The listing builds one solid part. Answer for the finished solid, in the listing's coordinates (mm). Face numbers are marked on the shaded views. A direction names the side the tool comes from. Round coordinates to 2 decimals unless told otherwise and drop trailing zeros. Write each loop counter-clockwise with the first axis right and the second up, starting at its lowest first coordinate (ties: lowest second). Pieces come first, ordered by that corner, then holes.
(1) Each of these flat-tipped pins is pushed along its axis until it touches: pin 1 Ø7.5 at (x, z) = (0, 0) entering from +Y; pin 2 Ø0.8 at (x, y) = (-10, 6) entering from +Z; pin 3 Ø0.8 at (y, z) = (5.5, 1) entering from -X; pin 4 Ø2 at (x, y) = (-7.5, 6) entering from -Z. Where does it stop, or does it pass through?
(2) A cutting plane is placed at C-C, the plane y = 2.75. Give the vertices of the cut face in (x, z) (3 decimals), and give its area (3 significant figures).
(3) A cutting plane is placed at A-A, the plane x = 0. Give the vertices of the cut face in (y, z) (3 decimals), and give its area (3 significant figures).
(4) Find the intervals of material crossed by probe 1 along X at (y, z) = (5.8, 0) (3 decimals); probe 2 along Z at (x, y) = (0, 5.3) (3 decimals); probe 3 along X at (y, z) = (4, -1), in increasing order.
(5) A cutting plane is placed at B-B, the plane z = 0. Give the vertices of the cut face in (x, y) (3 decimals), and give its area (3 significant figures).
(6) A cutting plane is placed at D-D, the plane z = -5.25. Give the vertices of the cut face in (x, y).
(7) For the marked faces 5, 6 and 7, determine the directions among +Z, -Z, +X, -X, +Y, -Y from which every point of the face is accessible in a straight line to the end or side of a thin tool.
(8) The mould has two halves that part along Z. Classify the marked faces 1, 2, 3 and 4: +Z half, -Z half, draft (parallel to the pull), parting line (faces both ways), or undercut.
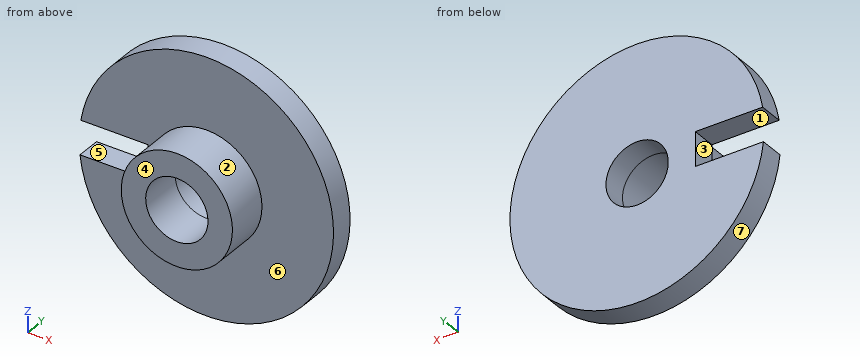
from build123d import *

# Parameters (mm, degrees)
SKETCH1_R           = 5.685
SKETCH1_R_2         = 3.185
BOSS_EXTRUDE1_DEPTH = 4.46
SKETCH2_R           = 13
BOSS_EXTRUDE2_DEPTH = 2.5
SKETCH3_R           = 3.185
CUT_EXTRUDE1_DEPTH  = 2.5
SKETCH4_W           = 8.515099108
SKETCH4_H           = 3.5
CUT_EXTRUDE2_DEPTH  = 10


with BuildPart() as part:
    # Sketch1 → Boss-Extrude1 (new body)
    with BuildSketch(Plane(origin=(0, 0, 0), x_dir=(1, 0, 0), z_dir=(0, 1, 0))):
        with Locations(Location((0, 0, 0), (0, 0, 270))):
            Circle(SKETCH1_R)
        with Locations(Location((0, 0, 0), (0, 0, 270))):
            Circle(SKETCH1_R_2, mode=Mode.SUBTRACT)
    extrude(amount=BOSS_EXTRUDE1_DEPTH)

    # Sketch2 → Boss-Extrude2 (add)
    with BuildSketch(Plane(origin=(0, 4.46, 0), x_dir=(1, 0, 0), z_dir=(0, 1, 0))):
        with Locations(Location((0, 0, 0), (0, 0, 270))):
            Circle(SKETCH2_R)
    extrude(amount=BOSS_EXTRUDE2_DEPTH)

    # Sketch3 → Cut-Extrude1 (cut)
    with BuildSketch(Plane.XZ.offset(-4.46)):
        with Locations(Location((0, 0, 0), (0, 0, 270))):
            Circle(SKETCH3_R)
    extrude(amount=-CUT_EXTRUDE1_DEPTH, mode=Mode.SUBTRACT)

    # Sketch4 → Cut-Extrude2 (cut)
    with BuildSketch(Plane.XZ.offset(-4.46)):
        with Locations((-10.213773727, 0.31798138)):
            Rectangle(SKETCH4_W, SKETCH4_H)
    extrude(amount=-CUT_EXTRUDE2_DEPTH, mode=Mode.SUBTRACT)


solid = part.part
Solutions:
1. pin 1: stops at y = 6.96
1. pin 2: stops at z = 8.77
1. pin 3: stops at x = -5.96
1. pin 4: stops at z = -11.26
2. outline: circle Ø11.37 at (0, 0); hole circle Ø6.37 at (0, 0)
2. area: 69.7 mm2
3. outline: (0, -5.685) - (4.46, -5.685) - (4.46, -13) - (6.96, -13) - (6.96, -3.185) - (0, -3.185) - close; (0, 3.185) - (6.96, 3.185) - (6.96, 13) - (4.46, 13) - (4.46, 5.685) - (0, 5.685) - close
3. area: 71.4 mm2
4. probe 1: x = -5.956 to -3.185, 3.185 to 13
4. probe 2: z = -13 to -3.185, 3.185 to 13
4. probe 3: x = -5.6 to -3.02, 3.02 to 5.6
5. outline: (-5.956, 4.46) - (-5.685, 4.46) - (-5.685, 0) - (-3.185, 0) - (-3.185, 6.96) - (-5.956, 6.96) - close; (3.185, 0) - (5.685, 0) - (5.685, 4.46) - (13, 4.46) - (13, 6.96) - (3.185, 6.96) - close
5. area: 53.8 mm2
6. outline: (-11.89, 4.46) - (-2.18, 4.46) - (-2.18, 0) - (2.18, 0) - (2.18, 4.46) - (11.89, 4.46) - (11.89, 6.96) - (-11.89, 6.96) - close
7. face 5: -X, +Y, -Y
7. face 6: -Y
7. face 7: +Y, -Y
8. face 1: undercut
8. face 2: parting line
8. face 3: undercut
8. face 4: draft
